from build123d import *

# Parameters (mm, degrees)
SKETCH2_R           = 19.8
BOSS_EXTRUDE1_DEPTH = 27
SKETCH3_R           = 14.5
BOSS_EXTRUDE2_DEPTH = 50
SKETCH5_R           = 1.6
CUT_EXTRUDE1_DEPTH  = 10
SKETCH6_R           = 6
BOSS_EXTRUDE3_DEPTH = 5.5
SKETCH7_R           = 3
BOSS_EXTRUDE4_DEPTH = 15


with BuildPart() as part:
    # Sketch2 → Boss-Extrude1 (new body)
    with BuildSketch(Plane.XY):
        Circle(SKETCH2_R)
    extrude(amount=BOSS_EXTRUDE1_DEPTH)

    # Sketch3 → Boss-Extrude2 (add)
    with BuildSketch(Plane.XY.offset(27)):
        Circle(SKETCH3_R)
    extrude(amount=BOSS_EXTRUDE2_DEPTH)

    # Sketch5 → Cut-Extrude1 (cut)
    with BuildSketch(Plane(origin=(0, 0, 0), x_dir=(-1, 0, 0), z_dir=(0, 0, -1))):
        with Locations((-15.5, 0)):
            Circle(SKETCH5_R)
        with Locations((7.75, 13.423393759)):
            Circle(SKETCH5_R)
        with Locations((7.75, -13.423393759)):
            Circle(SKETCH5_R)
    extrude(amount=-CUT_EXTRUDE1_DEPTH, mode=Mode.SUBTRACT)

    # Sketch6 → Boss-Extrude3 (add)
    with BuildSketch(Plane(origin=(0, 0, 0), x_dir=(-1, 0, 0), z_dir=(0, 0, -1))):
        with Locations(Location((0, 7, 0), (0, 0, 180))):
            Circle(SKETCH6_R)
    extrude(amount=BOSS_EXTRUDE3_DEPTH)

    # Sketch7 → Boss-Extrude4 (add)
    with BuildSketch(Plane(origin=(0, 0, -5.5), x_dir=(-1, 0, 0), z_dir=(0, 0, -1))):
        with Locations((0, 7)):
            Circle(SKETCH7_R)
    extrude(amount=BOSS_EXTRUDE4_DEPTH)


solid = part.part
Source: CAD feature listing. Evaluate the final solid. Frame: model axes, mm. A direction names the side the tool comes from. Give positions to 0.01 mm unless a question says otherwise; leave off trailing zeros. Order: outer loops, then holes, each group sorted by start corner. A loop starts at its lowest first (then second) coordinate and runs counter-clockwise, first axis right, second up. Notation, with made-up numbers: (5.5, 61.5) -> (11.5, 61.5) arc R33 cw to (11.5, 91.5) -> close; hole circle Ø11 at (37.25, 84). An arc over 180 degrees is marked (long way). Write item = value, one per line.
Q1. Cut plane C-C, the plane z = 15.5. Output: boundary loops of the cut face in (x, y), and give its area (3 significant figures).
Data:
outline = circle Ø39.6 at (0, 0)
area = 1,230 mm^2
Q2. Cut plane B-B, the plane x = 11. Output: boundary loops of the cut face in (y, z).
Data:
outline = (-16.46, 0) -> (16.46, 0) -> (16.46, 27) -> (9.45, 27) -> (9.45, 77) -> (-9.45, 77) -> (-9.45, 27) -> (-16.46, 27) -> close
Q3. Pull-direction query (X, two-part tool) for faces 4 (the face through (16, 0, 10)), 5 (the face through (-8, 13, 10)), 6 (the face through (0, 7, -20.5)), 7 (the face through (18.9, 5.9, 13.3)); classes: released by +X, released by -X, zero draft, split by the parting line, or undercut.
Data:
face_4 = undercut
face_5 = undercut
face_6 = zero draft
face_7 = split by the parting line
Q4. Pin query (flat end, axial travel): pin 1 (4 mm diameter, centred on x = -7.5, z = -5, fed in from -Y); pin 2 (1 mm diameter, centred on x = 1, z = 13, fed in from +Y); pin 3 (6 mm diameter, centred on x = 13, z = 29.5, fed in from -Y). Return the tip coordinate at first contact, or that it passes through.
Data:
pin_1 = 4.6
pin_2 = 19.79
pin_3 = -16.23
Q5. Set-up query: faces 1 (the face through (6.691, -12.864, 51.65)), 2 (the face through (0, 0, 77)), 3 (the face through (-8, -13, 10)). Return all of +Z, -Z, +X, -X, +Y, -Y with unobstructed straight access to the full face (end or side cutting, diameter ignored); none if empty.
Data:
face_1 = +Z
face_2 = +Z, +X, -X, +Y, -Y
face_3 = -Z
Q6. Cut plane D-D, the plane x = -7.75. Output: boundary loops of the cut face in (y, z).
Data:
outline = (-18.22, 0) -> (-15.02, 0) -> (-15.02, 10) -> (-11.82, 10) -> (-11.82, 0) -> (11.82, 0) -> (11.82, 10) -> (15.02, 10) -> (15.02, 0) -> (18.22, 0) -> (18.22, 27) -> (12.26, 27) -> (12.26, 77) -> (-12.26, 77) -> (-12.26, 27) -> (-18.22, 27) -> close
Q7. Cut plane A-A, the plane y = 0. Output: boundary loops of the cut face in (x, z), and give its area (3 significant figures).
Data:
outline = (-19.8, 0) -> (13.9, 0) -> (13.9, 10) -> (17.1, 10) -> (17.1, 0) -> (19.8, 0) -> (19.8, 27) -> (14.5, 27) -> (14.5, 77) -> (-14.5, 77) -> (-14.5, 27) -> (-19.8, 27) -> close
area = 2,490 mm^2
Q8. Material intervals for line 1 (Y direction, x = -7, z = 3); line 2 (Y direction, x = -7.75, z = 3.25); line 3 (Z direction, x = 12.5, y = 14.5), sorted ascending. Write a range as from..to.
Data:
line_1 = -18.52..-14.84, -12.01..12.01, 14.84..18.52
line_2 = -18.22..-15.02, -11.82..11.82, 15.02..18.22
line_3 = 0..27
